The listing builds one solid part. Answer for the finished solid, in the listing's coordinates (mm). Face numbers are marked on the shaded views. A direction names the side the tool comes from. Coordinates: 2 decimals unless noted, no trailing zeros. Loops run counter-clockwise (first coordinate to the right, second up) from the corner with the lowest first, then second, coordinate; pieces in that order, holes last. Notation, with made-up numbers: (-36.75, 48.25) - (-1.75, 48.25) arc R15 cw to (-1.75, 71.25) - close; hole circle Ø8 at (30, -4). An arc over 180 degrees is marked (long way). Write each question's results on one line, items separated by ' | '. Start each with the question number.
(1) For the marked faces 1, 2 and 3, determine the directions among +Z, -Z, +X, -X, +Y, -Y from which every point of the face is accessible in a straight line to the end or side of a thin tool.
(2) Consider line 1 (X direction, y = -8, z = 15.5); line 2 (X direction, y = -11.5, z = 0.5); line 3 (X direction, y = -11.5, z = 6). Determine where each line is inside the solid, lowest interval first. Write a range as from..to.
(3) Find section C-C on x = -4.5. Determine the outline of the cut face in (y, z).
(4) Find section B-B on y = -15.5. Determine the outline of the cut face in (x, z), then the cut area to 3 significant figures.
(5) Find section A-A on x = -11.5. Determine the outline of the cut face in (y, z).
(6) Given pin 1 Ø1 at (x, y) = (-4, 15.5) entering from +Z; pin 2 Ø3 at (x, y) = (-2.5, 7.5) entering from +Z; pin 3 Ø2 at (x, z) = (-17, 6.5) entering from +Y; pin 4 Ø4 at (x, z) = (-14, 0) entering from -Y, each flat-ended and moving along its own axis, determine where each tip first touches the part or whether it passes through.
from build123d import *

# Parameters (mm, degrees)
F2_R = 0.49999


# Not quite as in the source:
# - a fillet or chamfer is up to 0.001 mm smaller than in the source, because OpenCascade refuses the exact size


with BuildPart() as f1:
    # F0 (on Front) → F1 (revolve)
    with BuildSketch(Plane.XZ):
        Polygon((-20, 0), (0, 0), (0, 12.5), (-3, 12.5), (-3, 13.5), (-4, 13.5), (-4, 12.5), (-5, 12.5), (-5, 18), (-6.25, 18), (-6.25, 20), (-8.75, 20), (-8.75, 18), (-10, 18), (-10, 10), (-20, 10), align=None)
    revolve(axis=Axis((-10, 0, 0), (-1, 0, 0)))

    # F2 (radius 0.5 in the source; OpenCascade refuses exactly that, so slightly less here)
    f2_edges = [f1.edges().sort_by_distance(p)[0] for p in [
        (-20, 0, -10),
        (-3, 0, -13.5),
        (0, 0, -12.5),
        (-3, 0, -12.5),
        (-1.5, 0, 12.5),
    ]]
    fillet(f2_edges, radius=F2_R)


solid = f1.part
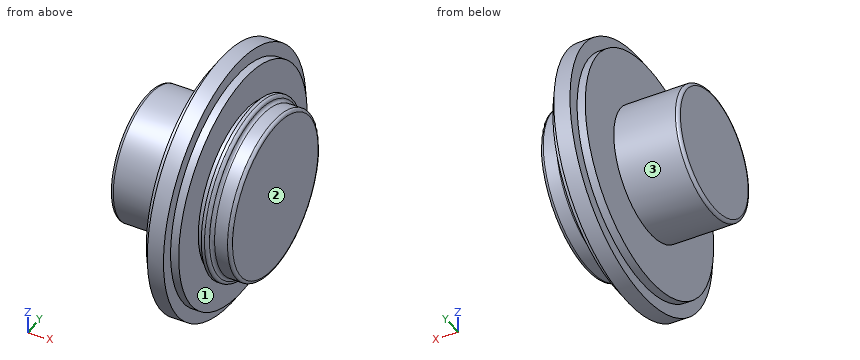
Values:
1) face 1: none | face 2: +Z, -Z, +X, +Y, -Y | face 3: -X
2) line 1: x = -10..-5 | line 2: x = -10..0 | line 3: x = -10..-5, -4..-3
3) outline: circle Ø25 at (0, 0)
4) outline: (-10, -9.15) - (-8.75, -9.15) - (-8.75, -12.64) - (-6.25, -12.64) - (-6.25, -9.15) - (-5, -9.15) - (-5, 9.15) - (-6.25, 9.15) - (-6.25, 12.64) - (-8.75, 12.64) - (-8.75, 9.15) - (-10, 9.15) - close | area: 109 mm²
5) outline: circle Ø20 at (0, 0)
6) pin 1: passes through | pin 2: stops at z = 11.93 | pin 3: stops at y = 8.35 | pin 4: stops at y = -10
